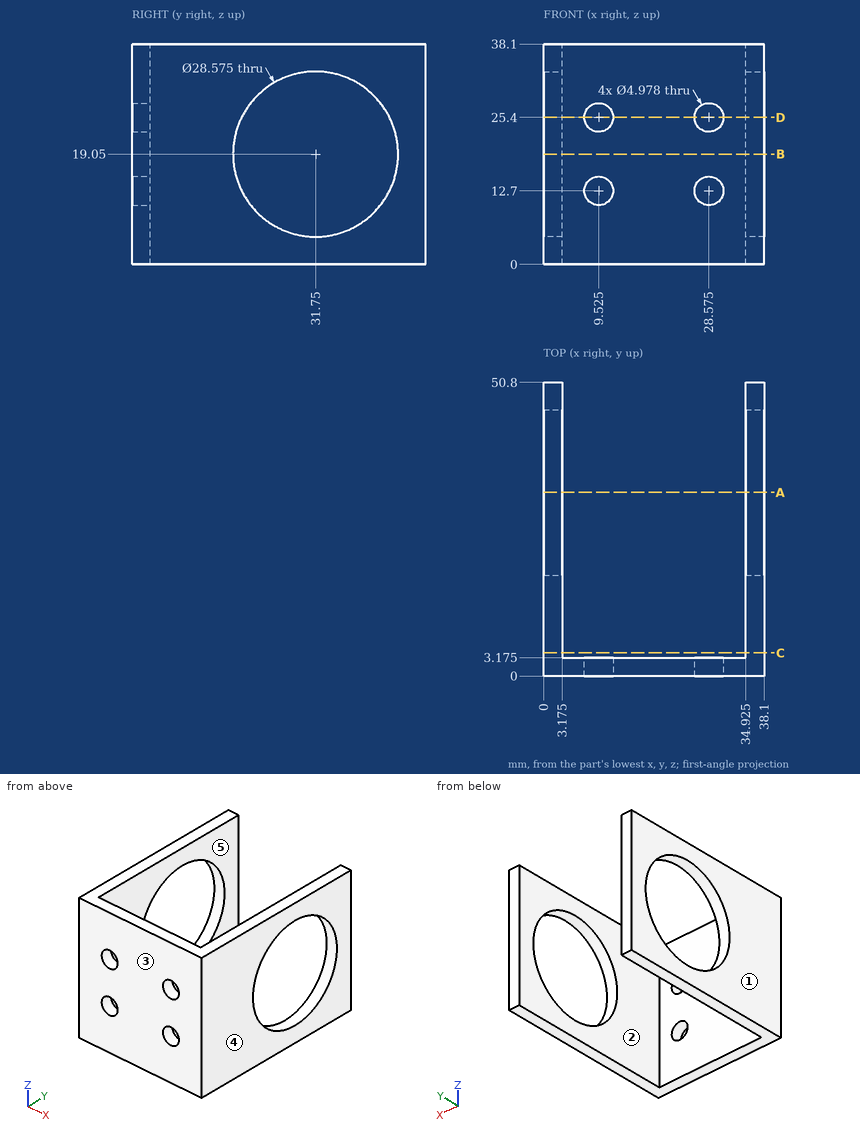
Here's the drawing with two shaded views (mm, measured from the low corner). I have some questions. A direction names the side the tool comes from. Give positions to 0.01 mm unless a question says otherwise; leave off trailing zeros. Loops run counter-clockwise (first coordinate to the right, second up) from the corner with the lowest first, then second, coordinate; pieces in that order, holes last. Notation, with made-up numbers: (48, -31) - (61, -31) arc R28 ccw to (61, -3) - close; hole circle Ø5 at (81, 51). An arc over 180 degrees is marked (long way). Answer in a Markdown table with one row per item. Add a question column.
Q1. Please list where these lines run through material, in increasing order: L1, parallel to X at y = 16, z = 8 (1 decimal); L2, parallel to Y at x = 36, z = 19; L3, parallel to Y at x = 14, z = 13 (1 decimal). Write a range as from..to.
Q2. If we section it at D-D (z = 25.4): List the corners of the cut face in (x, y) for me (1 decimal).
Q3. If we section it at B-B (z = 19.05): List the corners of the cut face in (x, y) for me (1 decimal).
Q4. We'd pull the mould along X, two halves only. Please class the marked faces 1, 2 and 3: +X half, -X half, draft (parallel to the pull), parting line (faces both ways), or undercut.
Q5. Which directions (+Z, -Z, +X, -X, +Y, -Y) give clear straight access to the entire face, cutting with the end or side of a thin tool? Please do the marked faces 4 and 5.
Q6. If we section it at A-A (y = 31.75): List the corners of the cut face in (x, z) for me (1 decimal).
Q7. For pin 1 (4.5 mm diameter, centred on x = 9.525, z = 25.4, fed in from +Y); pin 2 (8 mm diameter, centred on x = 28.575, z = 12.7, fed in from +Y) (3 decimals); pin 3 (3 mm diameter, centred on y = 27, z = 32.5, fed in from -X), each with a flat end and sliding along its axis, tell me the tip position at first contact or that it passes through.
Q8. If we section it at C-C (y = 4): List the corners of the cut face in (x, z) for me (1 decimal).
The answers:
| question | item | result |
|---|---|---|
| 1 | L1 | x = 0..3.2, 34.9..38.1 |
| 1 | L2 | y = 0..17.46, 46.04..50.8 |
| 1 | L3 | y = 0..3.2 |
| 2 | outline | (0, 0) - (7, 0) - (7, 3.2) - (3.2, 3.2) - (3.2, 19) - (0, 19) - close; (0, 44.5) - (3.2, 44.5) - (3.2, 50.8) - (0, 50.8) - close; (12, 0) - (26.1, 0) - (26.1, 3.2) - (12, 3.2) - close; (31.1, 0) - (38.1, 0) - (38.1, 19) - (34.9, 19) - (34.9, 3.2) - (31.1, 3.2) - close; (34.9, 44.5) - (38.1, 44.5) - (38.1, 50.8) - (34.9, 50.8) - close |
| 3 | outline | (0, 0) - (38.1, 0) - (38.1, 17.5) - (34.9, 17.5) - (34.9, 3.2) - (3.2, 3.2) - (3.2, 17.5) - (0, 17.5) - close; (0, 46) - (3.2, 46) - (3.2, 50.8) - (0, 50.8) - close; (34.9, 46) - (38.1, 46) - (38.1, 50.8) - (34.9, 50.8) - close |
| 4 | face 1 | -X half |
| 4 | face 2 | undercut |
| 4 | face 3 | draft |
| 5 | face 4 | +Z, -Z, +X, +Y, -Y |
| 5 | face 5 | +Z, -Z, +Y |
| 6 | outline | (0, 0) - (3.2, 0) - (3.2, 4.8) - (0, 4.8) - close; (0, 33.3) - (3.2, 33.3) - (3.2, 38.1) - (0, 38.1) - close; (34.9, 0) - (38.1, 0) - (38.1, 4.8) - (34.9, 4.8) - close; (34.9, 33.3) - (38.1, 33.3) - (38.1, 38.1) - (34.9, 38.1) - close |
| 7 | pin 1 | passes through |
| 7 | pin 2 | stops at y = 3.175 |
| 7 | pin 3 | stops at x = 0 |
| 8 | outline | (0, 0) - (3.2, 0) - (3.2, 38.1) - (0, 38.1) - close; (34.9, 0) - (38.1, 0) - (38.1, 38.1) - (34.9, 38.1) - close |
